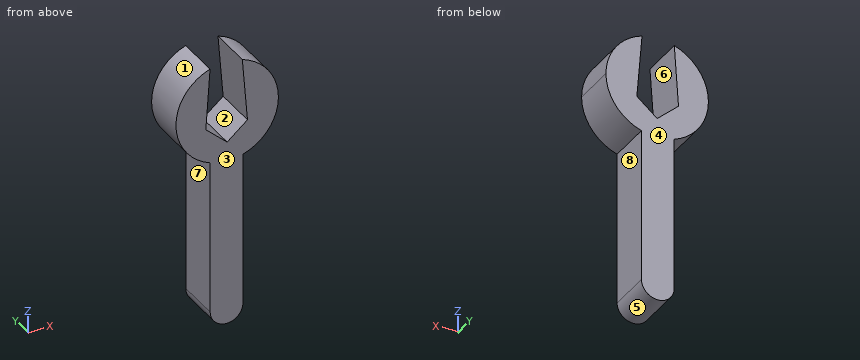
```python
from build123d import *

# Parameters (mm, degrees)
F1_DEPTH = 25.4


with BuildPart() as f1:
    # F0 (on Front) → F1 (new body)
    with BuildSketch(Plane.XZ):
        with BuildLine():
            ThreePointArc((8.776649, 21.15477), (23.105166, 31.531712), (28.580673, 48.354499))
            ThreePointArc((28.580673, 48.354499), (23.003939, 65.315443), (8.450032, 75.657462))
            Line((8.450032, 75.657462), (11.326279, 40.222812))
            Line((11.326279, 40.222812), (0, 30.639039))
            Line((0, 30.639039), (-11.907114, 41.094065))
            Line((-11.907114, 41.094065), (-9.546468, 75.293686))
            ThreePointArc((-9.546468, 75.293686), (-28.58065, 48.318335), (-9.478263, 21.391239))
            ThreePointArc((-9.478263, 21.391239), (-0.370196, 19.776224), (8.776649, 21.15477))
        make_face()
        with BuildLine():
            Line((8.776649, -64.327464), (8.776649, 21.15477))
            ThreePointArc((8.776649, 21.15477), (-0.370196, 19.776224), (-9.478263, 21.391239))
            Line((-9.478263, 21.391239), (-9.478263, -64.327464))
            ThreePointArc((-9.478263, -64.327464), (-0.350807, -73.45492), (8.776649, -64.327464))
        make_face()
    extrude(amount=F1_DEPTH)


solid = f1.part
```
Model file for the job. Use its own axes, mm. Face numbers are marked on the shaded views. A direction names the side the tool comes from. Coordinates: 2 decimals unless noted, no trailing zeros. Loops run counter-clockwise (first coordinate to the right, second up) from the corner with the lowest first, then second, coordinate; pieces in that order, holes last. Notation, with made-up numbers: (65, -37.5) - (101, -37.5) arc R12 cw to (101, -31.5) - close; hole circle Ø10 at (31, 41). An arc over 180 degrees is marked (long way). Answer as a JSON object with one key per item and string values. Group by question number.
(1) Probe line 1 along X through (y, z) = (-21.75, -10.5); line 2 along X through (y, z) = (-8, 61.5); line 3 along X through (y, z) = (-15.5, 47.5). List the from-to ranges inside material, lowest first.
(2) Cut at C-C (x = -15.5). Give the cut face in (y, z), then the cut area to 3 significant figures.
(3) Two-plate mould, pull along X, no slides. Class the marked faces 1, 2 and 3: released by +X, released by -X, zero draft, split by the parting line, or undercut.
(4) Cut at B-B (z = -53). Give the cut face in (x, y).
(5) Cut at A-A (y = -23.5). Give the cut face in (x, z).
(6) Tool access for the marked faces 4, 5, 6, 7 and 8: list every direction of +Z, -Z, +X, -X, +Y, -Y with a clear straight run to the whole face (end or side of a thin tool).
(7) Flat gauge pins, fed straight in: pin 1 (8 mm diameter, centred on x = -16.5, z = -19, fed in from +Y); pin 2 (12.5 mm diameter, centred on y = -8.5, z = -2, fed in from -X); pin 3 (12.5 mm diameter, centred on y = -11, z = -27.5, fed in from +X); pin 4 (1 mm diameter, centred on x = 14, y = -6, fed in from -Z). Where does each tip first touch, or does it go through?
Geometry says:
{
 "1": {"line 1": "x = -9.48 to 8.78", "line 2": "x = -25.38 to -10.5, 9.6 to 25.38", "line 3": "x = -28.57 to -11.46, 10.74 to 28.57"},
 "2": {"outline": "(-25.4, 24.34) - (0, 24.34) - (0, 72.37) - (-25.4, 72.37) - close", "area": "1,220 mm^2"},
 "3": {"face 1": "released by -X", "face 2": "undercut", "face 3": "zero draft"},
 "4": {"outline": "(-9.48, -25.4) - (8.78, -25.4) - (8.78, 0) - (-9.48, 0) - close"},
 "5": {"outline": "(-11.91, 41.09) - (-9.55, 75.29) arc R28.58 ccw to (-9.48, 21.39) - (-9.48, -64.33) arc R9.13 ccw to (8.78, -64.33) - (8.78, 21.15) arc R28.58 ccw to (28.58, 48.35) arc R28.58 ccw to (8.45, 75.66) - (11.33, 40.22) - (0, 30.64) - close"},
 "6": {"face 4": "+Z, -Z, +X, -X, +Y", "face 5": "-Z, +Y, -Y", "face 6": "+Y, -Y", "face 7": "-Z, -X, +Y, -Y", "face 8": "-Z, +X, +Y, -Y"},
 "7": {"pin 1": "passes through", "pin 2": "stops at x = -9.48", "pin 3": "stops at x = 8.78", "pin 4": "stops at z = 23.16"}
}
